Check sheet for the modelled part. Datum: model origin and axes. Units: mm. Face numbers are marked on the shaded views. A direction names the side the tool comes from. Round coordinates to 2 decimals unless told otherwise and drop trailing zeros. Order: outer loops, then holes, each group sorted by start corner. A loop starts at its lowest first (then second) coordinate and runs counter-clockwise, first axis right, second up.
Q1. Set-up check for the marked faces 4 and 5: record each of +Z, -Z, +X, -X, +Y, -Y from which the full face is reachable in a straight line by a thin tool's end or side.
Q2. Cross-section at D-D on z = 164. Record the cut outline in (x, y), then the cut area to 3 significant figures.
Q3. Mould release check, pull along Y, two halves, no side actions. Record for the marked faces 1, 2 and 3: +Y half, -Y half, draft (parallel to the pull), parting line (faces both ways), or undercut.
Q4. Depth check by flat-ended pin: P1, Ø1, axis at x = 3, y = 7, coming from the +Z side. Enter the tip coordinate at first touch or a pass-through.
Q5. Cross-section at A-A on y = 8. Record the cut outline in (x, z), then the cut area to 3 significant figures.
Q6. Cross-section at C-C on z = 81.5. Record the cut outline in (x, y), then the cut area to 3 significant figures.
Q7. Scan lines: probe 1 along X at (y, z) = (17.25, 127); probe 2 along Y at (x, z) = (24.6, 164). Record each from-to range of solid material in increasing order.
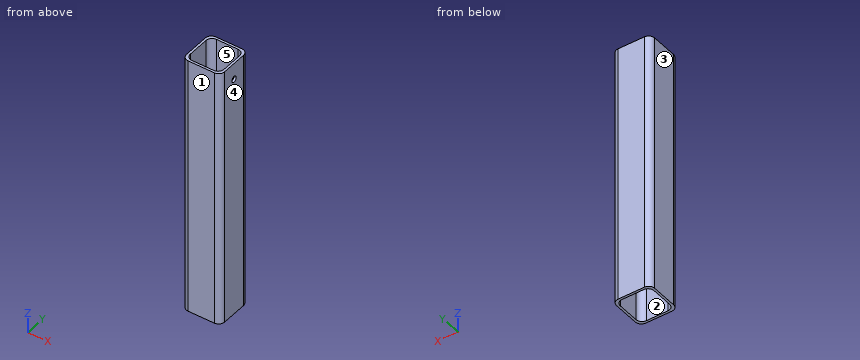
from build123d import *

# Parameters (mm, degrees)
SKETCH4_W           = 25.5
SKETCH4_H           = 25.5
SKETCH4_W_2         = 22.5
SKETCH4_H_2         = 22.5
BOSS_EXTRUDE1_DEPTH = 175
SKETCH5_R           = 2
CUT_EXTRUDE1_DEPTH  = 1.5
FILLET1_R           = 4


with BuildPart() as part:
    # Sketch4 → Boss-Extrude1 (new body)
    with BuildSketch(Plane.XY):
        with Locations((12.75, 12.75)):
            Rectangle(SKETCH4_W, SKETCH4_H)
        with Locations((12.75, 12.75)):
            Rectangle(SKETCH4_W_2, SKETCH4_H_2, mode=Mode.SUBTRACT)
    extrude(amount=BOSS_EXTRUDE1_DEPTH)

    # Sketch5 → Cut-Extrude1 (cut)
    with BuildSketch(Plane(origin=(25.5, 0, 0), x_dir=(0, 0, -1), z_dir=(1, 0, 0))):
        with Locations((-164, 12.75)):
            Circle(SKETCH5_R)
    extrude(amount=-CUT_EXTRUDE1_DEPTH, mode=Mode.SUBTRACT)

    # Fillet1
    fillet1_edges = [part.edges().sort_by_distance(p)[0] for p in [
        (1.5, 1.5, 87.5),
        (24, 1.5, 87.5),
        (24, 24, 87.5),
        (1.5, 24, 87.5),
        (0, 25.5, 87.5),
        (25.5, 25.5, 87.5),
        (25.5, 0, 87.5),
        (0, 0, 87.5),
    ]]
    fillet(fillet1_edges, radius=FILLET1_R)


solid = part.part
Results found:
1. face 4: +Z, -Z, +X, +Y, -Y
1. face 5: +Z, -Z
2. outline: (0, 4) arc R4 ccw to (4, 0) - (21.5, 0) arc R4 ccw to (25.5, 4) - (25.5, 10.75) - (24, 10.75) - (24, 5.5) arc R4 cw to (20, 1.5) - (5.5, 1.5) arc R4 cw to (1.5, 5.5) - (1.5, 20) arc R4 cw to (5.5, 24) - (20, 24) arc R4 cw to (24, 20) - (24, 14.75) - (25.5, 14.75) - (25.5, 21.5) arc R4 ccw to (21.5, 25.5) - (4, 25.5) arc R4 ccw to (0, 21.5) - close
2. area: 138 mm2
3. face 1: -Y half
3. face 2: undercut
3. face 3: draft
4. P1: passes through
5. outline: (0, 0) - (1.5, 0) - (1.5, 175) - (0, 175) - close; (24, 0) - (25.5, 0) - (25.5, 175) - (24, 175) - close
5. area: 525 mm2
6. outline: (0, 4) arc R4 ccw to (4, 0) - (21.5, 0) arc R4 ccw to (25.5, 4) - (25.5, 21.5) arc R4 ccw to (21.5, 25.5) - (4, 25.5) arc R4 ccw to (0, 21.5) - close; hole (1.5, 5.5) arc R4 ccw to (5.5, 1.5) - (20, 1.5) arc R4 ccw to (24, 5.5) - (24, 20) arc R4 ccw to (20, 24) - (5.5, 24) arc R4 ccw to (1.5, 20) - close
6. area: 144 mm2
7. probe 1: x = 0 to 1.5, 24 to 25.5
7. probe 2: y = 1.47 to 10.75, 14.75 to 24.03
